Design review of the part built by this model. Coordinates are the model's own, in mm. Give positions to 0.01 mm unless a question says otherwise; leave off trailing zeros. Loops run counter-clockwise (first coordinate to the right, second up) from the corner with the lowest first, then second, coordinate; pieces in that order, holes last. Notation, with made-up numbers: (64, -25.75) -> (70, -25.75) arc R26 cw to (70, 4.25) -> close; hole circle Ø2 at (-29.5, 56). An arc over 180 degrees is marked (long way). Use a Markdown table: item, result. Add a question column.
1. For pin 1 Ø3.5 at (x, y) = (-30.5, 10) entering from -Z, flat-tipped, find the tip position at first contact; note if it passes through.
2. Add section C-C (z = 0.2). Count the separate pieces of the cut face and the enclosed holes in it, and give its area (3 significant figures).
3. Add section A-A (y = 84). State the section outline as (x, z) points.
4. To check wall thickness, follow line 1 (Y direction, x = -9, z = 0.1); line 2 (Y direction, x = -11, z = 0.95) (3 decimals); line 3 (Y direction, x = 30.5, z = 0.45). State the ranges of each line that lie inside material, in increasing order.
5. Add section B-B (x = 5.5). State the section outline as (y, z) points.
```python
from build123d import *

# Parameters (mm, degrees)
SKETCH1_W                    = 82
SKETCH1_H                    = 208
BOSS_EXTRUDE1_DEPTH          = 1
F_3_0_3_DIAMETER_HOLE1_D     = 3
SKETCH7_W                    = 50
SKETCH7_H                    = 22
CUT_EXTRUDE1_DEPTH           = 10
F_1_75_1_75_DIAMETER_HOLE1_D = 1.75


with BuildPart() as part:
    # Sketch1 → Boss-Extrude1 (new body)
    with BuildSketch(Plane.XY):
        Rectangle(SKETCH1_W, SKETCH1_H)
    extrude(amount=BOSS_EXTRUDE1_DEPTH)

    # Ø3.0 (3) Diameter Hole1 (through all)
    with Locations(Plane.XY.offset(1)):
        with Locations((-30.5, 10), (30.5, 10), (30.5, -100), (-30.5, -100), (-30.5, 101.59999968), (30.5, 101.59999968), (30.5, -8.7), (-30.5, -8.7)):
            Hole(F_3_0_3_DIAMETER_HOLE1_D / 2)

    # Sketch7 → Cut-Extrude1 (cut)
    with BuildSketch(Plane(origin=(0, 0, 0), x_dir=(-1, 0, 0), z_dir=(0, 0, -1))):
        with Locations((-1, -22)):
            Rectangle(SKETCH7_W, SKETCH7_H)
        with Locations((-1, 88)):
            Rectangle(SKETCH7_W, SKETCH7_H)
    extrude(amount=-CUT_EXTRUDE1_DEPTH, mode=Mode.SUBTRACT)

    # Ø1.75 (1.75) Diameter Hole1 (through all)
    with Locations(Plane(origin=(0, 0, 0), x_dir=(-1, 0, 0), z_dir=(0, 0, -1))):
        with Locations((24.5, 0.65), (11, 0.65)):
            Hole(F_1_75_1_75_DIAMETER_HOLE1_D / 2)


solid = part.part
```
Taken from the geometry:
| question | item | result |
|---|---|---|
| 1 | pin 1 | stops at z = 0 |
| 2 | separate pieces | 1 |
| 2 | enclosed holes | 12 |
| 2 | area | 14,800 mm^2 |
| 3 | outline | (-41, 0) -> (-24, 0) -> (-24, 1) -> (-41, 1) -> close; (26, 0) -> (41, 0) -> (41, 1) -> (26, 1) -> close |
| 4 | line 1 | y = -104 to -33, -11 to 77, 99 to 104 |
| 4 | line 2 | y = -104 to -33, -11 to -0.225, 1.525 to 77, 99 to 104 |
| 4 | line 3 | y = -104 to -101.5, -98.5 to -10.2, -7.2 to 8.5, 11.5 to 100.1, 103.1 to 104 |
| 5 | outline | (-104, 0) -> (-33, 0) -> (-33, 1) -> (-104, 1) -> close; (-11, 0) -> (77, 0) -> (77, 1) -> (-11, 1) -> close; (99, 0) -> (104, 0) -> (104, 1) -> (99, 1) -> close |
